Check sheet for the drawn part. Datum: minimum x, y, z corner. Units: mm. A direction names the side the tool comes from. Give positions to 0.01 mm unless a question says otherwise; leave off trailing zeros. Loops run counter-clockwise (first coordinate to the right, second up) from the corner with the lowest first, then second, coordinate; pieces in that order, holes last. Notation, with made-up numbers: (65, 19) - (105, 19) arc R31 ccw to (105, 54) - close; hole circle Ø9 at (15.25, -9). An arc over 180 degrees is marked (long way). Use one line per item in the form item = value.
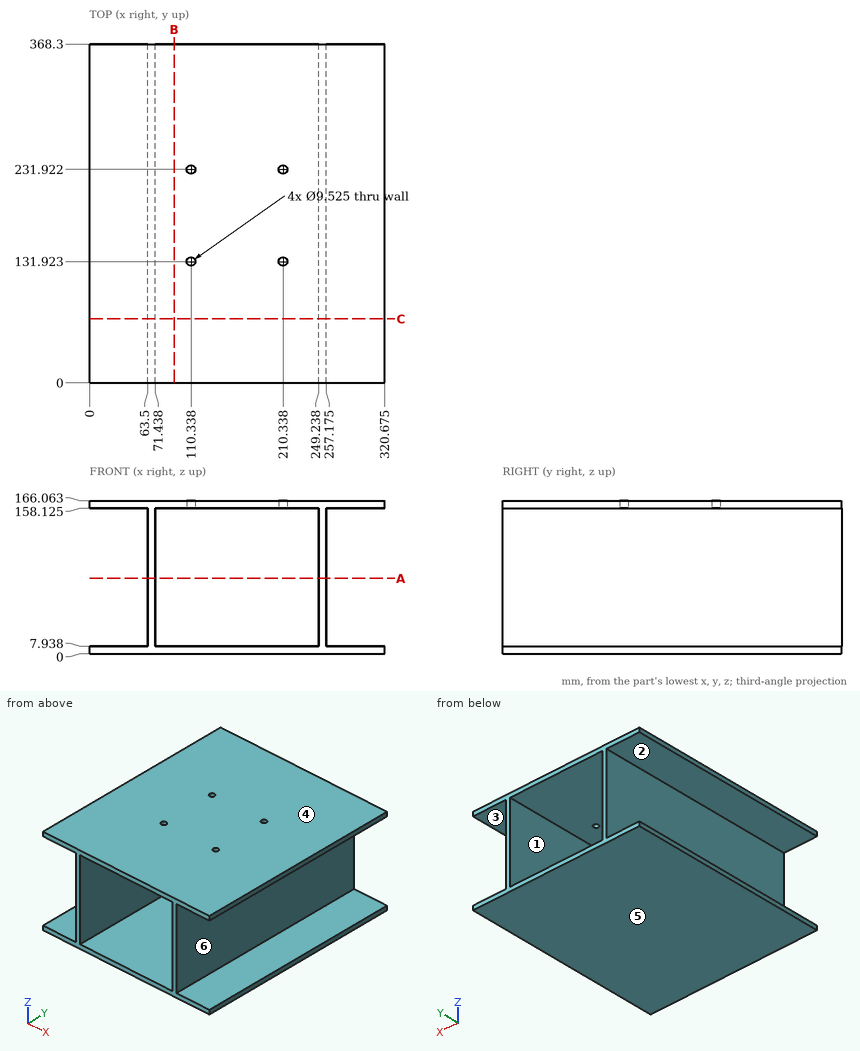
1. Draft check along Z on the marked faces 4, 5 and 6. Enter one of: released by +Z, released by -Z, zero draft, split by the parting line, or undercut.
Result set:
face_4 = released by +Z
face_5 = released by -Z
face_6 = undercut
2. Tool access check on the marked faces 1, 2 and 3. Record the directions out of +Z, -Z, +X, -X, +Y, -Y that give a thin tool (end or side, any length) a straight path to the whole face; none if there is none.
Result set:
face_1 = +Y, -Y
face_2 = -X, +Y, -Y
face_3 = +X, +Y, -Y
3. Depth check by flat-ended pin: pin 1 Ø10 at (y, z) = (289, 131.5) entering from +X (1 decimal). Enter the tip coordinate at first touch or a pass-through.
Result set:
pin_1 = 257.2
4. Scan lines: probe 1 along X at (y, z) = (38.5, 148.5) (1 decimal); probe 2 along Z at (x, y) = (237, 264) (1 decimal). Record each from-to range of solid material in increasing order.
Result set:
probe_1 = 63.5 to 71.4, 249.2 to 257.2
probe_2 = 0 to 7.9, 158.1 to 166.1
5. Section check B-B, the plane x = 92. Record the cut outline in (y, z) (1 decimal).
Result set:
outline = (0, 0) - (368.3, 0) - (368.3, 7.9) - (0, 7.9) - close; (0, 158.1) - (368.3, 158.1) - (368.3, 166.1) - (0, 166.1) - close
6. Section check C-C, the plane y = 69.5. Record the cut outline in (x, z) (1 decimal).
Result set:
outline = (0, 0) - (320.7, 0) - (320.7, 7.9) - (257.2, 7.9) - (257.2, 158.1) - (320.7, 158.1) - (320.7, 166.1) - (0, 166.1) - (0, 158.1) - (63.5, 158.1) - (63.5, 7.9) - (0, 7.9) - close; hole (71.4, 7.9) - (249.2, 7.9) - (249.2, 158.1) - (71.4, 158.1) - close
7. Section check A-A, the plane z = 82. Record the cut outline in (x, y) (1 decimal).
Result set:
outline = (63.5, 0) - (71.4, 0) - (71.4, 368.3) - (63.5, 368.3) - close; (249.2, 0) - (257.2, 0) - (257.2, 368.3) - (249.2, 368.3) - close
